from build123d import *

# Parameters (mm, degrees)
CROQUIS1_R              = 1.5
SALIENTE_EXTRUIR1_DEPTH = 3
CROQUIS2_W              = 4
CROQUIS2_H              = 26
SALIENTE_EXTRUIR2_DEPTH = 62.8
SALIENTE_EXTRUIR3_DEPTH = 26
CROQUIS5_W              = 40.3
CROQUIS5_H              = 21
CROQUIS5_R              = 1.5
CORTAR_EXTRUIR1_DEPTH   = 26


with BuildPart() as part:
    # Croquis1 → Saliente-Extruir1 (new body)
    with BuildSketch(Plane.XY):
        with BuildLine():
            Line((-20.5, -13), (22, -13))
            Line((22, -13), (22, 13))
            Line((22, 13), (-20.5, 13))
            ThreePointArc((-20.5, 13), (-21.560660172, 12.560660172), (-22, 11.5))
            Line((-22, 11.5), (-22, -11.5))
            ThreePointArc((-22, -11.5), (-21.560660172, -12.560660172), (-20.5, -13))
        make_face()
        with Locations((-6.61, 0)):
            Circle(CROQUIS1_R, mode=Mode.SUBTRACT)
        with Locations((-13.61, 0)):
            Circle(CROQUIS1_R, mode=Mode.SUBTRACT)
        with Locations((-6.61, 7)):
            Circle(CROQUIS1_R, mode=Mode.SUBTRACT)
        with Locations((0.39, 0)):
            Circle(CROQUIS1_R, mode=Mode.SUBTRACT)
        with Locations((-6.61, -7)):
            Circle(CROQUIS1_R, mode=Mode.SUBTRACT)
    extrude(amount=SALIENTE_EXTRUIR1_DEPTH)

    # Croquis2 → Saliente-Extruir2 (add)
    with BuildSketch(Plane.XY.offset(3)):
        with Locations((20, 0)):
            Rectangle(CROQUIS2_W, CROQUIS2_H)
    extrude(amount=SALIENTE_EXTRUIR2_DEPTH)

    # Croquis3 → Saliente-Extruir3 (add)
    with BuildSketch(Plane.XZ.offset(13)):
        Polygon((18, 3), (18, 4.5), (16.5, 3), align=None)
    extrude(amount=-SALIENTE_EXTRUIR3_DEPTH)

    # Croquis5 → Cortar-Extruir1 (cut)
    with BuildSketch(Plane.ZY.offset(-18)):
        with Locations((38.1664, 0)):
            Rectangle(CROQUIS5_W, CROQUIS5_H)
        with Locations(Location((14.5, -5, 0), (0, 0, 270))):
            Circle(CROQUIS5_R)
        with Locations(Location((14.5164, 5, 0), (0, 0, 270))):
            Circle(CROQUIS5_R)
        with Locations(Location((61.8164, 5, 0), (0, 0, 270))):
            Circle(CROQUIS5_R)
        with Locations(Location((61.8328, -5, 0), (0, 0, 270))):
            Circle(CROQUIS5_R)
    extrude(amount=-CORTAR_EXTRUIR1_DEPTH, mode=Mode.SUBTRACT)


solid = part.part
Build history of the part. All positions in model axes, mm. A direction names the side the tool comes from. Coordinates: 2 decimals unless noted, no trailing zeros. Order: outer loops, then holes, each group sorted by start corner. A loop starts at its lowest first (then second) coordinate and runs counter-clockwise, first axis right, second up. Notation, with made-up numbers: (-32, 36.25) - (-23, 36.25) arc R36 ccw to (-23, 72.25) - close; hole circle Ø11 at (23.5, 47.25). An arc over 180 degrees is marked (long way). Write item = value, one per line. Start each with the question number.
1) Saw through at B-B on x = 0.39. Write the cut outline in (y, z), then the cut area to 3 significant figures.
2) Saw through at C-C on z = 57.5. Write the cut outline in (x, y).
3) Saw through at A-A on y = 9.5. Write the cut outline in (x, z), then the cut area to 3 significant figures.
4) Two-plate mould, pull along Y, no slides. Class faces 4 (the face through (20, 0, 18.016)), 5 (the face through (20, -13, 23)), 6 (the face through (22, -0.2, 17.8)): pulls with the +Y half, pulls with the -Y half, needs draft (parallel to the pull), parting line crosses it, or undercut.
5) 3-axis set-ups, long thin cutter, end or side, ignore diameter. For faces 1 (the face through (-3, 0, 3)), 2 (the face through (-0.8, -0.91, 1.48)), 3 (the face through (20, 0, 58.316)): which of +Z, -Z, +X, -X, +Y, -Y reach the whole face in a straight line?
6) Wall check: line 1 along Z through (x, y) = (19.8, 5); line 2 along Z through (x, y) = (19, -8.75); line 3 along Y through (x, z) = (20, 14). Give the ranges that are in metal, low to high. Write a range as from..to.
7) Flat gauge pins, fed straight in: pin 1 Ø2.5 at (x, y) = (-13.61, 0) entering from -Z; pin 2 Ø5 at (x, y) = (-6.61, 7) entering from +Z; pin 3 Ø4 at (y, z) = (-5, 14.5) entering from -X. Where does each tip first touch, or does it go through?
8) Saw through at D-D on x = -6.61. Write the cut outline in (y, z).
From the geometry:
q1.outline = (-13, 0) - (-1.5, 0) - (-1.5, 3) - (-13, 3) - close; (1.5, 0) - (13, 0) - (13, 3) - (1.5, 3) - close
q1.area = 69.0 mm^2
q2.outline = (18, -13) - (22, -13) - (22, -10.5) - (18, -10.5) - close; (18, 10.5) - (22, 10.5) - (22, 13) - (18, 13) - close
q3.outline = (-22, 0) - (22, 0) - (22, 18.02) - (18, 18.02) - (18, 4.5) - (16.5, 3) - (-22, 3) - close; (18, 58.32) - (22, 58.32) - (22, 65.8) - (18, 65.8) - close
q3.area = 223 mm^2
q4.face_4 = undercut
q4.face_5 = pulls with the -Y half
q4.face_6 = needs draft
q5.face_1 = +Z, -X, +Y, -Y
q5.face_2 = +Z, -Z
q5.face_3 = +X, -X
q6.line_1 = 0..13.02, 16.02..18.02, 58.32..60.32, 63.32..65.8
q6.line_2 = 0..18.02, 58.32..65.8
q6.line_3 = -13..-6.41, -3.59..3.59, 6.41..13
q7.pin_1 = through
q7.pin_2 = 3
q7.pin_3 = 18
q8.outline = (-13, 0) - (-8.5, 0) - (-8.5, 3) - (-13, 3) - close; (-5.5, 0) - (-1.5, 0) - (-1.5, 3) - (-5.5, 3) - close; (1.5, 0) - (5.5, 0) - (5.5, 3) - (1.5, 3) - close; (8.5, 0) - (13, 0) - (13, 3) - (8.5, 3) - close
